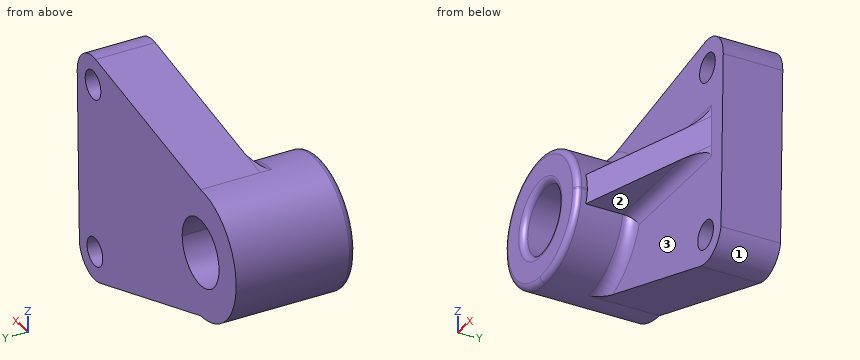
```python
from build123d import *

# Parameters (mm, degrees)
F1_DEPTH     = 12.7
F2_DEPTH     = 25.4
F3_R         = 3.0339595682
F4_DEPTH     = 25.4
F5_R         = 1.2264204897
F7_DEPTH     = 3.175
F8_T4_ANGLE  = 97.0773840638
F8_T9_DEPTH  = 34.7132171162
F8_T14_ANGLE = 97.0773840638
F8_T19_DEPTH = 34.7132171162


# Not quite as in the source:
# - a fillet or chamfer that OpenCascade refuses, or shapes differently, is made with other operations: its cross-section is extruded or revolved along the edge and cut away or added


with BuildPart() as f1:
    # F0 (on Front) → F1 (new body)
    with BuildSketch(Plane.XZ):
        with BuildLine():
            ThreePointArc((0, -13.789825828), (9.6376295499, -9.8628288552), (13.7861481364, -0.3184586768))
            ThreePointArc((13.7861481364, -0.3184586768), (13.7889063745, -0.1592399559), (13.789825828, 0))
            ThreePointArc((13.789825828, 0), (9.7508793544, 9.7508793544), (0, 13.789825828))
            ThreePointArc((0, 13.789825828), (-13.789825828, 0), (0, -13.789825828))
        make_face()
        with BuildLine():
            ThreePointArc((7.1353728529, -0.1648264167), (-7.1368004494, 0.0824187037), (7.137276336, 0))
            ThreePointArc((7.137276336, 0), (7.1368004494, -0.0824187037), (7.1353728529, -0.1648264167))
        make_face(mode=Mode.SUBTRACT)
        with BuildLine():
            ThreePointArc((13.789825828, 0), (13.7889063745, -0.1592399559), (13.7861481364, -0.3184586768))
            ThreePointArc((13.7861481364, -0.3184586768), (9.6376295499, -9.8628288552), (0, -13.789825828))
            Line((0, -13.789825828), (38.9815755188, -27.3394305259))
            ThreePointArc((38.9815755188, -27.3394305259), (43.9885292005, -26.9000346666), (46.9867042389, -22.8659795937))
            Line((46.9867042389, -22.8659795937), (47.8485122544, 14.4418842975))
            ThreePointArc((47.8485122544, 14.4418842975), (45.7311207367, 19.22142423), (40.6978976177, 20.6335197794))
            Line((40.6978976177, 20.6335197794), (0, 13.789825828))
            ThreePointArc((0, 13.789825828), (9.7508793544, 9.7508793544), (13.789825828, 0))
        make_face()
    extrude(amount=F1_DEPTH)

    # F0 (on Front) → F2 (join)
    with BuildSketch(Plane.XZ):
        with BuildLine():
            ThreePointArc((0, -13.789825828), (9.6376295499, -9.8628288552), (13.7861481364, -0.3184586768))
            ThreePointArc((13.7861481364, -0.3184586768), (13.7889063745, -0.1592399559), (13.789825828, 0))
            ThreePointArc((13.789825828, 0), (9.7508793544, 9.7508793544), (0, 13.789825828))
            ThreePointArc((0, 13.789825828), (-13.789825828, 0), (0, -13.789825828))
        make_face()
        with BuildLine():
            ThreePointArc((7.1353728529, -0.1648264167), (-7.1368004494, 0.0824187037), (7.137276336, 0))
            ThreePointArc((7.137276336, 0), (7.1368004494, -0.0824187037), (7.1353728529, -0.1648264167))
        make_face(mode=Mode.SUBTRACT)
    extrude(amount=F2_DEPTH)

    # F3 (on face) → F4 (cut)
    with BuildSketch(Plane.XZ.offset(12.7)):
        with Locations((40.9957959094, -21.5446131849)):
            Circle(F3_R)
        with Locations((41.715248914, 14.5835620822)):
            Circle(F3_R)
    extrude(amount=-F4_DEPTH, mode=Mode.SUBTRACT)

    # F5
    f5_edges = [f1.edges().sort_by_distance(p)[0] for p in [
        (0, -25.4, 13.789826),
        (-7.137276, -25.4, 0),
    ]]
    fillet(f5_edges, radius=F5_R)

    # F6 (on Top) → F7 (join, symmetric)
    with BuildSketch(Plane.XY):
        Polygon((13.3344670758, -12.2673781589), (13.3344670758, -23.1246650219), (44.4674044847, -12.2673781589), align=None)
    extrude(amount=F7_DEPTH, both=True)

    # F8: fillet of radius 2.4528409794 on 4 edges, made by hand


with BuildPart() as f8_tool2:
    # F8_s3 → F8_t4 (revolve)
    with BuildSketch(Plane(origin=(0, 0, 0), x_dir=(0, 1, 0), z_dir=(0.0543746304, 0, 0.9985206055))):
        with BuildLine():
            ThreePointArc((-15.1528409794, -13.789825828), (-13.4184204897, -14.5082463177), (-12.7, -16.2426668074))
            Line((-12.7, -16.2426668074), (-12.6509431804, -16.2426668074))
            Line((-12.6509431804, -16.2426668074), (-12.6509431804, -13.7407690084))
            Line((-12.6509431804, -13.7407690084), (-15.1528409794, -13.7407690084))
            Line((-15.1528409794, -13.7407690084), (-15.1528409794, -13.789825828))
        make_face()
    revolve(axis=Axis((0, -12.7, 0), (0, 1, 0)), revolution_arc=F8_T4_ANGLE)

    split(bisect_by=Plane(origin=(-4.2765210661, 0, -12.3033499954), x_dir=(0, 1, 0), z_dir=(0.3283216608, 0, 0.9445659781)), keep=Keep.TOP)


with BuildPart() as f1_1:
    add(f1.part)

    # F8_t1: union F8_tool2
    add(f8_tool2.part)


with BuildPart() as f8_tool7:
    # F8_s8 → F8_t9 (new body)
    with BuildSketch(Plane.YZ.offset(45.6797155903)):
        with BuildLine():
            ThreePointArc((-12.7, -5.6278409794), (-13.4184204897, -3.8934204897), (-15.1528409794, -3.175))
            Line((-15.1528409794, -3.175), (-15.1528409794, -3.1259431804))
            Line((-15.1528409794, -3.1259431804), (-12.6509431804, -3.1259431804))
            Line((-12.6509431804, -3.1259431804), (-12.6509431804, -5.6278409794))
            Line((-12.6509431804, -5.6278409794), (-12.7, -5.6278409794))
        make_face()
    extrude(amount=-F8_T9_DEPTH)

    split(bisect_by=Plane(origin=(8.6359194604, -24.7632344453, 0), x_dir=(0, 0, 1), z_dir=(-0.3292899537, 0.9442288528, 0)), keep=Keep.TOP)


with BuildPart() as f1_2:
    add(f1_1.part)

    # F8_t6: union F8_tool7
    add(f8_tool7.part)


with BuildPart() as f8_tool12:
    # F8_s13 → F8_t14 (revolve)
    with BuildSketch(Plane(origin=(0, 0, 0), x_dir=(0, 1, 0), z_dir=(-0.9842130406, 0, -0.1769878264))):
        with BuildLine():
            ThreePointArc((-15.1528409794, -13.789825828), (-13.4184204897, -14.5082463177), (-12.7, -16.2426668074))
            Line((-12.7, -16.2426668074), (-12.6509431804, -16.2426668074))
            Line((-12.6509431804, -16.2426668074), (-12.6509431804, -13.7407690084))
            Line((-12.6509431804, -13.7407690084), (-15.1528409794, -13.7407690084))
            Line((-15.1528409794, -13.7407690084), (-15.1528409794, -13.789825828))
        make_face()
    revolve(axis=Axis((0, -12.7, 0), (0, 1, 0)), revolution_arc=F8_T14_ANGLE)

    split(bisect_by=Plane(origin=(-2.2551070217, 0, 13.4106106059), x_dir=(0, 1, 0), z_dir=(0.1658301489, 0, -0.9861543296)), keep=Keep.TOP)


with BuildPart() as f1_3:
    add(f1_2.part)

    # F8_t11: union F8_tool12
    add(f8_tool12.part)


with BuildPart() as f8_tool17:
    # F8_s18 → F8_t19 (new body)
    with BuildSketch(Plane.YZ.offset(45.6797155903)):
        with BuildLine():
            ThreePointArc((-12.7, 5.6278409794), (-13.4184204897, 3.8934204897), (-15.1528409794, 3.175))
            Line((-15.1528409794, 3.175), (-15.1528409794, 3.1259431804))
            Line((-15.1528409794, 3.1259431804), (-12.6509431804, 3.1259431804))
            Line((-12.6509431804, 3.1259431804), (-12.6509431804, 5.6278409794))
            Line((-12.6509431804, 5.6278409794), (-12.7, 5.6278409794))
        make_face()
    extrude(amount=-F8_T19_DEPTH)

    split(bisect_by=Plane(origin=(8.6359194604, -24.7632344453, 0), x_dir=(0, 0, 1), z_dir=(-0.3292899537, 0.9442288528, 0)), keep=Keep.TOP)


with BuildPart() as f1_4:
    add(f1_3.part)

    # F8_t16: union F8_tool17
    add(f8_tool17.part)


solid = f1_4.part
```
CAD build for the part. Positions are in the model's coordinates, mm. Face numbers are marked on the shaded views. A direction names the side the tool comes from. Round coordinates to 2 decimals unless told otherwise and drop trailing zeros. Order: outer loops, then holes, each group sorted by start corner. A loop starts at its lowest first (then second) coordinate and runs counter-clockwise, first axis right, second up.
Item 1: Pin check, flat tips, straight feed: pin 1 (2 mm diameter, centred on y = -20.5, z = 13.5, fed in from +X); pin 2 (21.5 mm diameter, centred on x = 33, z = 0.5, fed in from -Y); pin 3 (4 mm diameter, centred on x = 19.5, z = -10.5, fed in from -Y); pin 4 (3 mm diameter, centred on x = -4.5, z = -1.5, fed in from -Y). Stop position of each tip, or through.
Item 2: Saw through at B-B on y = -4.25. Write the cut outline in (x, z), then the cut area to 3 significant figures.
Item 3: Saw through at C-C on y = -17.25. Write the cut outline in (x, z) (3 decimals), then the cut area to 3 significant figures.
Item 4: Tool access for the marked faces 1, 2 and 3: list every direction of +Z, -Z, +X, -X, +Y, -Y with a clear straight run to the whole face (end or side of a thin tool).
Item 5: Saw through at A-A on x = 42.5. Write the cut outline in (y, z) (3 decimals), then the cut area to 3 significant figures.
Item 6: Saw through at D-D on x = 20. Write the cut outline in (y, z) (3 decimals).
Item 7: Probe line 1 along Z through (x, y) = (0, -22); line 2 along Z through (x, y) = (43.5, -3.75); line 3 along Y through (x, z) = (18.5, -9). List the from-to ranges inside material, lowest first.
Reported:
1. pin 1: stops at x = 5.82
1. pin 2: stops at y = -20.02
1. pin 3: stops at y = -12.7
1. pin 4: passes through
2. outline: (0, -13.79) - (38.98, -27.34) arc R6.13 ccw to (46.99, -22.87) - (47.85, 14.44) arc R6.13 ccw to (40.7, 20.63) - (0, 13.79) arc R13.79 ccw to start; hole circle Ø14.27 at (0, 0); hole circle Ø6.07 at (41, -21.54); hole circle Ø6.07 at (41.72, 14.58)
2. area: 1,940 mm2
3. outline: (13.419, -3.175) - (30.18, -3.175) - (30.18, 3.175) - (13.419, 3.175) arc R13.79 ccw (long way) to start; hole circle Ø14.275 at (0, 0)
3. area: 542 mm2
4. face 1: -Z, +Y, -Y
4. face 2: -Z, +X, -Y
4. face 3: +X, -Y
5. outline: (-12.953, -4.542) arc R2.453 cw to (-12.7, -5.628) - (-12.7, -18.91) - (0, -18.91) - (0, 11.653) - (-12.7, 11.653) - (-12.7, 5.628) arc R2.453 cw to (-12.953, 4.542) - close; (-12.7, -27.492) - (0, -27.492) - (0, -24.179) - (-12.7, -24.179) - close; (-12.7, 17.514) - (0, 17.514) - (0, 20.668) - (-12.7, 20.668) - close
5. area: 473 mm2
6. outline: (-20.8, -3.175) - (-15.153, -3.175) arc R2.453 cw to (-12.7, -5.628) - (-12.7, -20.742) - (0, -20.742) - (0, 17.153) - (-12.7, 17.153) - (-12.7, 5.628) arc R2.453 cw to (-15.153, 3.175) - (-20.8, 3.175) - close
7. line 1: z = -13.79 to -7.14, 7.14 to 13.79
7. line 2: z = -27.15 to -23.26, -19.83 to 12.13, 17.04 to 20.45
7. line 3: y = -12.7 to 0
